For this review, take the finished solid that the model builds, in its own axes (mm). A direction names the side the tool comes from. Give positions to 0.01 mm unless a question says otherwise; leave off trailing zeros. Write each loop counter-clockwise with the first axis right and the second up, starting at its lowest first coordinate (ties: lowest second). Pieces come first, ordered by that corner, then holes. Notation, with made-up numbers: M 52,-15 L 63,-15 A5 ccw 63,-8 Z; hole C -9,45 d8. An arc over 180 degrees is marked long. Use one line per item in the form item = value. Start each with the question number.
Q1. Consider section D-D on y = 5.75. Write out the cut boundary in (x, z), and give its area (3 significant figures).
Q2. Consider section B-B on y = 22.5. Write out the cut boundary in (x, z).
Q3. Consider section C-C on x = 79. Write out the cut boundary in (y, z).
Q4. Clearance check with flat-ended pins moving along their axes: pin 1 Ø0.9 at (x, z) = (86, 1) entering from +Y; pin 2 Ø0.9 at (x, z) = (86, 2) entering from -Y. State where each tip first meets the part, or that it passes through.
Q5. Consider section A-A on x = 15. Write out the cut boundary in (y, z).
Q6. Tool access review of faces 4 (the flat face through (85, 7, 1)), 5 (the cylindrical face through (15.46, 21.61, 1.48)): name each direction out of +Z, -Z, +X, -X, +Y, -Y from which nothing blocks a thin tool from reaching the whole face with its end or side.
Q7. Mouldability with a two-part tool opening along Y and no side actions: class faces 1 (the flat face through (85, 25, 1)), 2 (the cylindrical face through (54.263, 27.676, 1.479)), 3 (the flat face through (86, 20, 1)) as released by +Y, released by -Y, zero draft, split by the parting line, or undercut.
Q8. For probe 1 along Y at (x, z) = (67, 1.6); probe 2 along X at (y, z) = (9.5, 1.5); probe 3 along Y at (x, z) = (19.5, 1), list the stretches that pass through material, from the lowest coordinate up. Write a range as [from, to].
```python
from build123d import *

# Parameters (mm, degrees)
SKETCH1_R           = 1.5
SKETCH1_R_2         = 1
BOSS_EXTRUDE1_DEPTH = 3
FILLET1_R           = 5


with BuildPart() as part:
    # Sketch1 → Boss-Extrude1 (new body)
    with BuildSketch(Plane.XY):
        Polygon((85, 30), (85, 20), (88, 20), (88, 10), (85, 10), (85, 3), (75, 3), (75, 0), (0, 0), (0, 30), align=None)
        with Locations((15, 15)):
            Circle(SKETCH1_R, mode=Mode.SUBTRACT)
        with Locations((7.5, 15)):
            Circle(SKETCH1_R_2, mode=Mode.SUBTRACT)
        with Locations((9.696699141, 20.303300859)):
            Circle(SKETCH1_R_2, mode=Mode.SUBTRACT)
        with Locations((15, 22.5)):
            Circle(SKETCH1_R_2, mode=Mode.SUBTRACT)
        with Locations((20.303300859, 20.303300859)):
            Circle(SKETCH1_R_2, mode=Mode.SUBTRACT)
        with Locations((22.5, 15)):
            Circle(SKETCH1_R_2, mode=Mode.SUBTRACT)
        with Locations((20.303300859, 9.696699141)):
            Circle(SKETCH1_R_2, mode=Mode.SUBTRACT)
        with Locations((15, 7.5)):
            Circle(SKETCH1_R_2, mode=Mode.SUBTRACT)
        with Locations((9.696699141, 9.696699141)):
            Circle(SKETCH1_R_2, mode=Mode.SUBTRACT)
        with Locations((82, 27)):
            Circle(SKETCH1_R_2, mode=Mode.SUBTRACT)
        with Locations((79, 27)):
            Circle(SKETCH1_R_2, mode=Mode.SUBTRACT)
        with Locations((76, 27)):
            Circle(SKETCH1_R_2, mode=Mode.SUBTRACT)
        with Locations((73, 27)):
            Circle(SKETCH1_R_2, mode=Mode.SUBTRACT)
        with Locations((70, 27)):
            Circle(SKETCH1_R_2, mode=Mode.SUBTRACT)
        with Locations((67, 27)):
            Circle(SKETCH1_R_2, mode=Mode.SUBTRACT)
        with Locations((64, 27)):
            Circle(SKETCH1_R_2, mode=Mode.SUBTRACT)
        with Locations((61, 27)):
            Circle(SKETCH1_R_2, mode=Mode.SUBTRACT)
        with Locations((58, 27)):
            Circle(SKETCH1_R_2, mode=Mode.SUBTRACT)
        with Locations((55, 27)):
            Circle(SKETCH1_R_2, mode=Mode.SUBTRACT)
        with Locations((52, 27)):
            Circle(SKETCH1_R_2, mode=Mode.SUBTRACT)
        with Locations((49, 27)):
            Circle(SKETCH1_R_2, mode=Mode.SUBTRACT)
        with Locations((46, 27)):
            Circle(SKETCH1_R_2, mode=Mode.SUBTRACT)
        with Locations((43, 27)):
            Circle(SKETCH1_R_2, mode=Mode.SUBTRACT)
        with Locations((40, 27)):
            Circle(SKETCH1_R_2, mode=Mode.SUBTRACT)
    extrude(amount=BOSS_EXTRUDE1_DEPTH)

    # Fillet1
    fillet1_edges = [part.edges().sort_by_distance(p)[0] for p in [
        (0, 0, 1.5),
        (0, 30, 1.5),
    ]]
    fillet(fillet1_edges, radius=FILLET1_R)


solid = part.part
```
Working result:
q1.outline = M 0,0 L 85,0 L 85,3 L 0,3 Z
q1.area = 255 mm²
q2.outline = M 0,0 L 14,0 L 14,3 L 0,3 Z; M 16,0 L 85,0 L 85,3 L 16,3 Z
q3.outline = M 3,0 L 26,0 L 26,3 L 3,3 Z; M 28,0 L 30,0 L 30,3 L 28,3 Z
q4.pin_1 = 20
q4.pin_2 = 10
q5.outline = M 0,0 L 6.5,0 L 6.5,3 L 0,3 Z; M 8.5,0 L 13.5,0 L 13.5,3 L 8.5,3 Z; M 16.5,0 L 21.5,0 L 21.5,3 L 16.5,3 Z; M 23.5,0 L 30,0 L 30,3 L 23.5,3 Z
q6.face_4 = +Z, -Z, +X, -Y
q6.face_5 = +Z, -Z
q7.face_1 = zero draft
q7.face_2 = undercut
q7.face_3 = released by +Y
q8.probe_1 = [0, 26], [28, 30]
q8.probe_2 = [0, 8.72], [10.68, 19.32], [21.28, 85]
q8.probe_3 = [0, 9.1], [10.29, 19.71], [20.9, 30]
